from build123d import *

# Parameters (mm, degrees)
SKETCH1_W           = 51.5
SKETCH1_H           = 59
BOSS_EXTRUDE1_DEPTH = 29
SKETCH2_W           = 7.5
SKETCH2_H           = 24.5
BOSS_EXTRUDE3_DEPTH = 8.2
SKETCH7_R           = 1.5
CUT_EXTRUDE1_DEPTH  = 8.2
SKETCH8_R           = 1.5
BOSS_EXTRUDE4_DEPTH = 2


with BuildPart() as part:
    # Sketch1 → Boss-Extrude1 (new body)
    with BuildSketch(Plane.XY):
        with Locations((25.75, 29.5)):
            Rectangle(SKETCH1_W, SKETCH1_H)
    extrude(amount=BOSS_EXTRUDE1_DEPTH)

    # Sketch2 → Boss-Extrude3 (add)
    with BuildSketch(Plane(origin=(0, 59, 0), x_dir=(1, 0, 0), z_dir=(0, 1, 0))):
        with Locations((9.75, -14.5)):
            Rectangle(SKETCH2_W, SKETCH2_H)
    boss_extrude3 = extrude(amount=BOSS_EXTRUDE3_DEPTH)

    # Sketch7 → Cut-Extrude1 (cut)
    with BuildSketch(Plane.ZY.offset(-6)):
        with Locations((6.75, 63.2)):
            Circle(SKETCH7_R)
        with Locations((22.25, 63.2)):
            Circle(SKETCH7_R)
    cut_extrude1 = extrude(amount=-CUT_EXTRUDE1_DEPTH, mode=Mode.SUBTRACT)

    # Mirror3: Boss-Extrude3, Cut-Extrude1 across plane
    add(boss_extrude3.mirror(Plane.ZX.offset(29.5)))
    add(cut_extrude1.mirror(Plane.ZX.offset(29.5)), mode=Mode.SUBTRACT)

    # Sketch8 → Boss-Extrude4 (add)
    with BuildSketch(Plane.ZY):
        with Locations((14.5, 43.7)):
            Circle(SKETCH8_R)
    extrude(amount=BOSS_EXTRUDE4_DEPTH)


solid = part.part
Design review of the part built by this model. Coordinates are the model's own, in mm. A direction names the side the tool comes from. Round coordinates to 2 decimals unless told otherwise and drop trailing zeros. Write each loop counter-clockwise with the first axis right and the second up, starting at its lowest first coordinate (ties: lowest second). Pieces come first, ordered by that corner, then holes. Notation, with made-up numbers: (86.25, 66.5) -> (122.25, 66.5) arc R31 cw to (122.25, 100.5) -> close; hole circle Ø4 at (-35, -4). An arc over 180 degrees is marked (long way). One line per question, with ' | ' between items.
(1) Take a section at B-B, the plane y = 63.2. State the section outline as (x, z) points.
Result sheet:
outline: (6, 2.25) -> (13.5, 2.25) -> (13.5, 5.25) -> (6, 5.25) -> close; (6, 8.25) -> (13.5, 8.25) -> (13.5, 20.75) -> (6, 20.75) -> close; (6, 23.75) -> (13.5, 23.75) -> (13.5, 26.75) -> (6, 26.75) -> close
(2) Take a section at D-D, the plane z = 19.75. State the section outline as (x, y) points, and give its area (3 significant figures).
Result sheet:
outline: (0, 0) -> (6, 0) -> (6, -8.2) -> (13.5, -8.2) -> (13.5, 0) -> (51.5, 0) -> (51.5, 59) -> (13.5, 59) -> (13.5, 67.2) -> (6, 67.2) -> (6, 59) -> (0, 59) -> close | area: 3,160 mm2
(3) Take a section at C-C, the plane x = 9.5. State the section outline as (y, z) points.
Result sheet:
outline: (-8.2, 2.25) -> (0, 2.25) -> (0, 0) -> (59, 0) -> (59, 2.25) -> (67.2, 2.25) -> (67.2, 26.75) -> (59, 26.75) -> (59, 29) -> (0, 29) -> (0, 26.75) -> (-8.2, 26.75) -> close; hole circle Ø3 at (-4.2, 6.75); hole circle Ø3 at (-4.2, 22.25); hole circle Ø3 at (63.2, 6.75); hole circle Ø3 at (63.2, 22.25)
(4) Draft analysis for pull direction Z (two halves, no side actions). For faces 4 (the flat face through (10, -4, 2.25)), 5 (the flat face through (13.5, -4, 15)), 6 (the cylindrical face through (9.7, 62.29, 21.06)), state which applies: released by +Z, released by -Z, zero draft, split by the parting line, or undercut.
Result sheet:
face 4: released by -Z | face 5: zero draft | face 6: undercut
(5) Wall thickness on line 1 (Z direction, x = 9, y = -4); line 2 (Y direction, x = 9, z = 6.75); line 3 (Y direction, x = 38.5, z = 14.5): over which ranges is each line inside the solid? List them lowest first. Write a range as [from, to].
Result sheet:
line 1: [2.25, 5.26], [8.24, 20.76], [23.74, 26.75] | line 2: [-8.2, -5.7], [-2.7, 61.7], [64.7, 67.2] | line 3: [0, 59]
(6) Machinability: for faces 1 (the cylindrical face through (-0.99, 44.71, 13.39)), 2 (the flat face through (13.5, 63, 15)), 3 (the flat face through (10, 63, 26.75)), which of the approach directions +Z, -Z, +X, -X, +Y, -Y give a long, thin tool a straight path to every point of the face, cutting with its end or side? Answer none if there is none.
Result sheet:
face 1: -X | face 2: +Z, -Z, +X, +Y | face 3: +Z, +X, -X, +Y
(7) Take a section at A-A, the plane z = 6.75. State the section outline as (x, y) points.
Result sheet:
outline: (0, 0) -> (6, 0) -> (6, -2.7) -> (13.5, -2.7) -> (13.5, 0) -> (51.5, 0) -> (51.5, 59) -> (13.5, 59) -> (13.5, 61.7) -> (6, 61.7) -> (6, 59) -> (0, 59) -> close; (6, -8.2) -> (13.5, -8.2) -> (13.5, -5.7) -> (6, -5.7) -> close; (6, 64.7) -> (13.5, 64.7) -> (13.5, 67.2) -> (6, 67.2) -> close
(8) Insertion check: P1, Ø4, axis at y = 63.2, z = 6.75, coming from the +X side; P2, Ø14.5, axis at x = 35.5, z = 14, coming from the -Y side; P3, Ø1, axis at y = 30.5, z = 22.5, coming from the -X side; P4, Ø6, axis at x = 9, y = 61.5, coming from the +Z side. Each pin has a flat end and moves straight along its axis. Give the tip position at first contact, or say it passes through.
Result sheet:
P1: x = 13.5 | P2: y = 0 | P3: x = 0 | P4: z = 29
